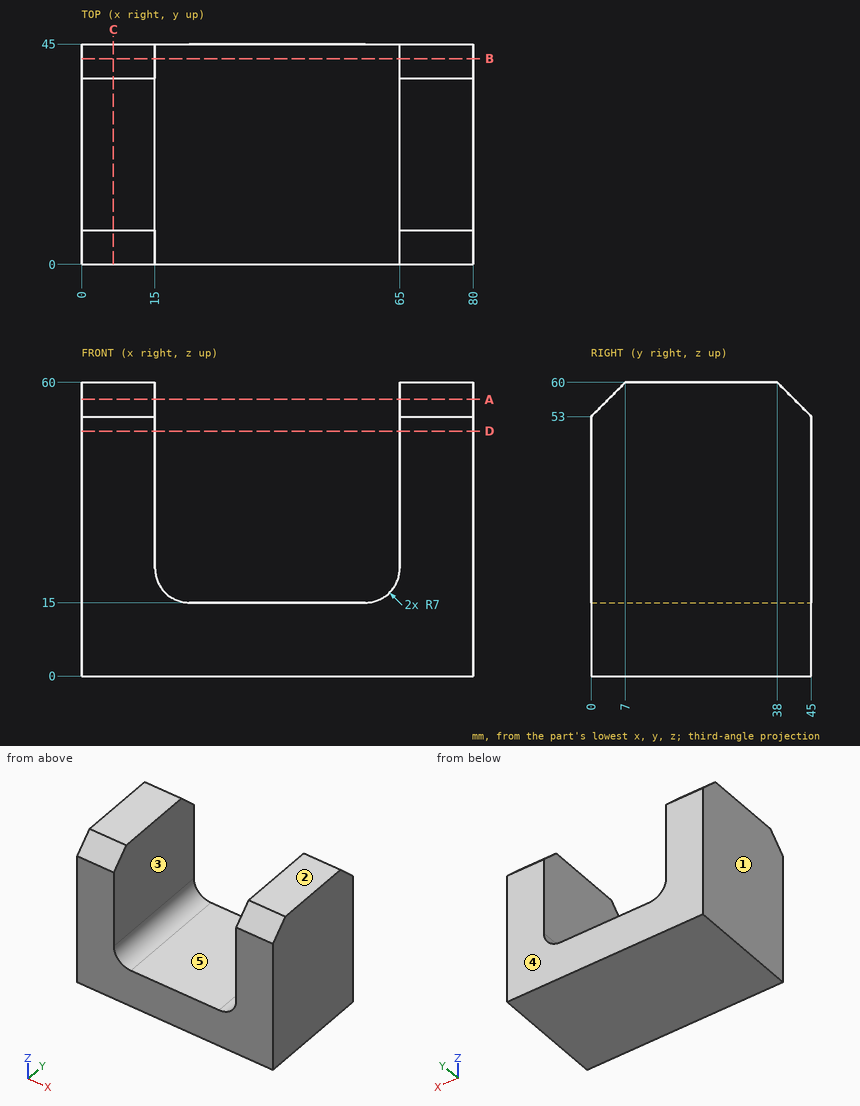
Input: dimensioned drawing with shaded views. Units: mm. Origin: part minimum x, y, z. A direction names the side the tool comes from. Give positions to 0.01 mm unless a question says otherwise; leave off trailing zeros. Write each loop counter-clockwise with the first axis right and the second up, starting at its lowest first coordinate (ties: lowest second). Pieces come first, ordered by that corner, then holes.
1. First-contact query: pin 1 (18 mm diameter, centred on x = 47, y = 21.5, fed in from +Z). Flat tip, straight axial feed; report the tip coordinate or a pass-through.
2. Section query C-C (x = 6.5). Return the cut outline in (y, z).
3. Pull-direction query (X, two-part tool) for the marked faces 1, 2 and 3; classes: +X half, -X half, draft (parallel to the pull), parting line (faces both ways), or undercut.
4. Section query A-A (z = 56.5). Return the cut outline in (x, y), then the cut area to 3 significant figures.
5. Section query B-B (y = 42). Return the cut outline in (x, z), then the cut area to 3 significant figures.
6. Material intervals for line 1 along X through (y, z) = (25, 37.5); line 2 along Z through (x, y) = (53, 25); line 3 along X through (y, z) = (41.5, 21), sorted ascending.
7. Access query for the marked faces 4 and 5. Directions: +Z, -Z, +X, -X, +Y, -Y. A direction counts if a zero-diameter tool reaches every point of the face in a straight line with its end or side. Return the directions, or none.
8. Section query D-D (z = 50). Return the cut outline in (x, y).
Output values:
1. pin 1: stops at z = 15
2. outline: (0, 0) - (45, 0) - (45, 53) - (38, 60) - (7, 60) - (0, 53) - close
3. face 1: -X half
3. face 2: draft
3. face 3: undercut
4. outline: (0, 3.5) - (15, 3.5) - (15, 41.5) - (0, 41.5) - close; (65, 3.5) - (80, 3.5) - (80, 41.5) - (65, 41.5) - close
4. area: 1,140 mm2
5. outline: (0, 0) - (80, 0) - (80, 56) - (65, 56) - (65, 22) arc R7 cw to (58, 15) - (22, 15) arc R7 cw to (15, 22) - (15, 56) - (0, 56) - close
5. area: 2,450 mm2
6. line 1: x = 0 to 15, 65 to 80
6. line 2: z = 0 to 15
6. line 3: x = 0 to 15.07, 64.93 to 80
7. face 4: +Z, -Z, +X, -X, +Y
7. face 5: +Z, +Y, -Y
8. outline: (0, 0) - (15, 0) - (15, 45) - (0, 45) - close; (65, 0) - (80, 0) - (80, 45) - (65, 45) - close
